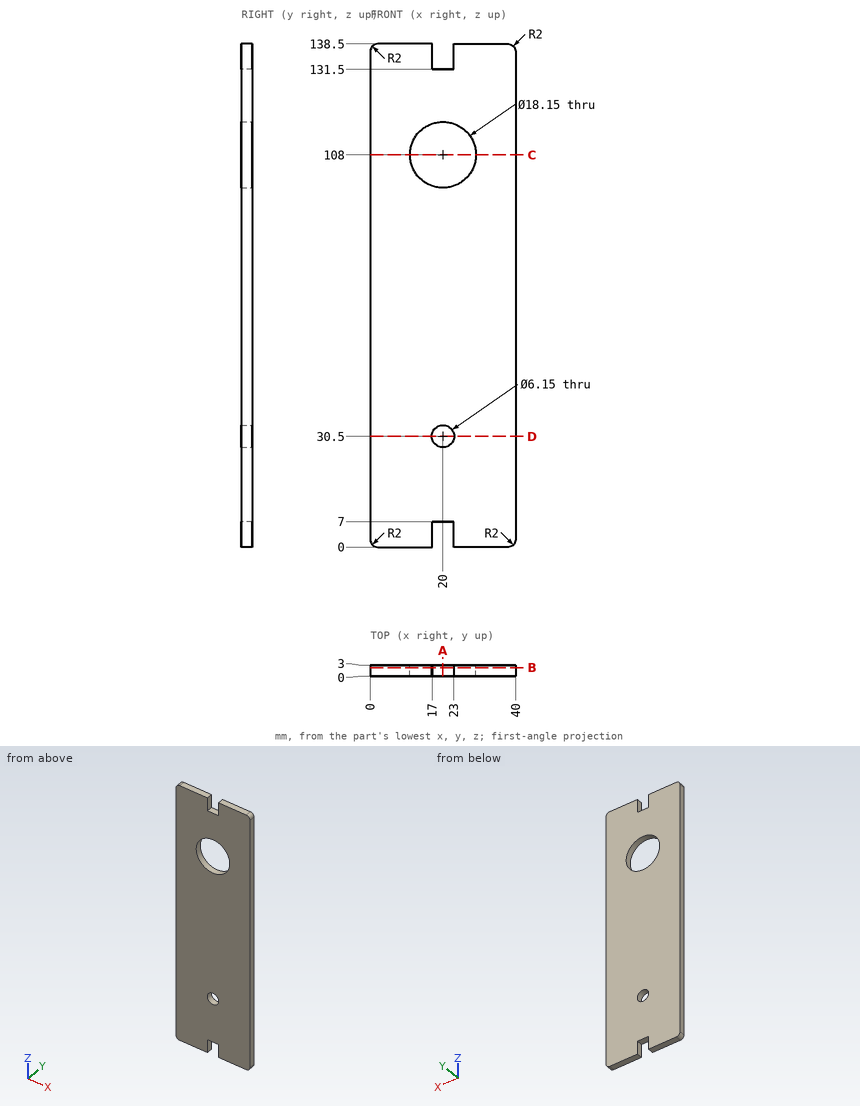
Source: three-view drawing plus pictorial views. Frame: mm from the lowest corner of the part. Give positions to 0.01 mm unless a question says otherwise; leave off trailing zeros. Write each loop counter-clockwise with the first axis right and the second up, starting at its lowest first coordinate (ties: lowest second). Pieces come first, ordered by that corner, then holes. Notation, with made-up numbers: (20.5, 53) - (29.5, 53) arc R25 cw to (29.5, 68) - close; hole circle Ø8 at (-12, 5.25). An arc over 180 degrees is marked (long way). Write item = value, one per line. Start each with the question number.
Q1. Pin query (flat end, axial travel): pin 1 Ø1.5 at (x, y) = (22, 1.5) entering from -Z; pin 2 Ø1.5 at (x, y) = (21.5, 2) entering from +Z; pin 3 Ø14.5 at (x, z) = (20, 108) entering from -Y. Return the tip coordinate at first contact, or that it passes through.
Q2. Cut plane B-B, the plane y = 2.3. Return loops of the section in (x, z) (3 decimals), then the cut area to 3 significant figures.
Q3. Cut plane C-C, the plane z = 108. Return loops of the section in (x, y) (3 decimals), then the cut area to 4 significant figures.
Q4. Cut plane D-D, the plane z = 30.5. Return loops of the section in (x, y) (3 decimals).
Q5. Material intervals for probe 1 along Z at (x, y) = (20, 1.85) (3 decimals); probe 2 along Z at (x, y) = (21, 1.8); probe 3 along Z at (x, y) = (25, 0.4), sorted ascending.
Q6. Cut plane A-A, the plane x = 20. Return loops of the section in (y, z) (3 decimals), then the cut area to 3 significant figures.
Computed values:
q1.pin_1 = 7
q1.pin_2 = 131.5
q1.pin_3 = through
q2.outline = (0, 2) arc R2 ccw to (2, 0) - (17, 0) - (17, 7) - (23, 7) - (23, 0) - (38, 0) arc R2 ccw to (40, 2) - (40, 136.5) arc R2 ccw to (38, 138.5) - (23, 138.5) - (23, 131.5) - (17, 131.5) - (17, 138.5) - (2, 138.5) arc R2 ccw to (0, 136.5) - close; hole circle Ø18.15 at (20, 108); hole circle Ø6.15 at (20, 30.5)
q2.area = 5,160 mm²
q3.outline = (0, 0) - (10.925, 0) - (10.925, 3) - (0, 3) - close; (29.075, 0) - (40, 0) - (40, 3) - (29.075, 3) - close
q3.area = 65.55 mm²
q4.outline = (0, 0) - (16.925, 0) - (16.925, 3) - (0, 3) - close; (23.075, 0) - (40, 0) - (40, 3) - (23.075, 3) - close
q5.probe_1 = 7 to 27.425, 33.575 to 98.925, 117.075 to 131.5
q5.probe_2 = 7 to 27.59, 33.41 to 98.98, 117.02 to 131.5
q5.probe_3 = 0 to 100.43, 115.57 to 138.5
q6.outline = (0, 7) - (3, 7) - (3, 27.425) - (0, 27.425) - close; (0, 33.575) - (3, 33.575) - (3, 98.925) - (0, 98.925) - close; (0, 117.075) - (3, 117.075) - (3, 131.5) - (0, 131.5) - close
q6.area = 301 mm²
